The model under review builds one solid part; all positions refer to its coordinate system, in mm. Face numbers are marked on the shaded views. A direction names the side the tool comes from. Coordinates: 2 decimals unless noted, no trailing zeros. Loops run counter-clockwise (first coordinate to the right, second up) from the corner with the lowest first, then second, coordinate; pieces in that order, holes last. Notation, with made-up numbers: (13, 57.5) - (63, 57.5) arc R16 ccw to (63, 67.5) - close; hole circle Ø8 at (82, 21.5). An arc over 180 degrees is marked (long way). Answer in a Markdown table with one row per item. Add a question column.
(1) Machinability: for the marked faces 3, 4 and 5, which of the approach directions +Z, -Z, +X, -X, +Y, -Y give a long, thin tool a straight path to every point of the face, cutting with its end or side? Answer none if there is none.
(2) We need section D-D on y = -13. Write out the cut boundary in (x, z), plus the area to 3 significant figures.
(3) We need section C-C on z = 3.5. Write out the cut boundary in (x, y).
(4) We need section A-A on y = 0.75. Write out the cut boundary in (x, z), plus the area to 3 significant figures.
(5) We need section B-B on x = -0.5. Write out the cut boundary in (y, z), plus the area to 3 significant figures.
(6) For line 1 along X through (y, z) = (-14, 0); line 2 along X through (y, z) = (-1.65, 0) (3 decimals), list the stretches that pass through material, from the lowest coordinate up.
(7) For P1, Ø0.9, axis at x = -0.5, z = 2, coming from the +Y side; P2, Ø1.3, axis at x = 0.5, z = 1, coming from the +Y side; P3, Ø3, axis at y = -13, z = -3, coming from the -X side; P4, Ø0.5, axis at x = -1.5, z = 1.5, coming from the -Y side, all flat-tipped, find the tip position at first contact; note any pin that passes through.
(8) Mouldability with a two-part tool opening along Z and no side actions: class the marked faces 1 and 2 as +Z half, -Z half, draft (parallel to the pull), parting line (faces both ways), or undercut.
from build123d import *

# Parameters (mm, degrees)
SKETCH1_R           = 5
SKETCH1_R_2         = 2.6
BOSS_EXTRUDE1_DEPTH = 8
BOSS_EXTRUDE2_START = 6
SKETCH2_R           = 5
SKETCH2_R_2         = 2.175
BOSS_EXTRUDE2_DEPTH = 6
BOSS_EXTRUDE3_START = 1.5
SKETCH3_R           = 5
BOSS_EXTRUDE3_DEPTH = 1.5
BOSS_EXTRUDE4_START = 13
SKETCH4_R           = 5
BOSS_EXTRUDE4_DEPTH = 13


with BuildPart() as part:
    # Sketch1 → Boss-Extrude1 (new body)
    # profile 1 of 6: a face of its own
    with BuildSketch(Plane(origin=(0, 0, 0), x_dir=(1, 0, 0), z_dir=(0, 1, 0))):
        with Locations(Location((0, 0, 0), (0, 0, 270))):
            Circle(SKETCH1_R)
        Circle(SKETCH1_R_2, mode=Mode.SUBTRACT)
    # profile 2 of 6: a face of its own
    with BuildSketch(Plane(origin=(0, 0, 0), x_dir=(1, 0, 0), z_dir=(0, 1, 0))):
        with BuildLine():
            Line((2.111719424, 1.51678643), (2.095106807, -1.539651735))
            ThreePointArc((2.095106807, -1.539651735), (2.470554361, -0.810161188), (2.6, 0))
            ThreePointArc((2.6, 0), (2.474921262, 0.796721249), (2.111719424, 1.51678643))
        make_face()
    # profile 3 of 6: a face of its own
    with BuildSketch(Plane(origin=(0, 0, 0), x_dir=(1, 0, 0), z_dir=(0, 1, 0))):
        with BuildLine():
            ThreePointArc((-0.816872207, -2.468343533), (0.789992429, -2.477077303), (2.095106807, -1.539651735))
            Line((2.095106807, -1.539651735), (-0.816872207, -2.468343533))
        make_face()
    # profile 4 of 6: a face of its own
    with BuildSketch(Plane(origin=(0, 0, 0), x_dir=(1, 0, 0), z_dir=(0, 1, 0))):
        with BuildLine():
            ThreePointArc((-2.599961596, 0.014131536), (-2.111719424, -1.51678643), (-0.816872207, -2.468343533))
            Line((-0.816872207, -2.468343533), (-2.599961596, 0.014131536))
        make_face()
    # profile 5 of 6: a face of its own
    with BuildSketch(Plane(origin=(0, 0, 0), x_dir=(1, 0, 0), z_dir=(0, 1, 0))):
        with BuildLine():
            Line((-2.599961596, 0.014131536), (-0.789992429, 2.477077303))
            ThreePointArc((-0.789992429, 2.477077303), (-2.095106807, 1.539651735), (-2.599961596, 0.014131536))
        make_face()
    # profile 6 of 6: a face of its own
    with BuildSketch(Plane(origin=(0, 0, 0), x_dir=(1, 0, 0), z_dir=(0, 1, 0))):
        with BuildLine():
            Line((-0.789992429, 2.477077303), (2.111719424, 1.51678643))
            ThreePointArc((2.111719424, 1.51678643), (0.816872207, 2.468343533), (-0.789992429, 2.477077303))
        make_face()
    extrude(amount=BOSS_EXTRUDE1_DEPTH)

    # Sketch2 → Boss-Extrude2 (add)
    with BuildSketch(Plane.XZ.offset(BOSS_EXTRUDE2_START)):
        with Locations(Location((0, 0, 0), (0, 0, 270))):
            Circle(SKETCH2_R)
        with Locations(Location((0, 0, 0), (0, 0, 87.049070531))):
            Circle(SKETCH2_R_2, mode=Mode.SUBTRACT)
    extrude(amount=-BOSS_EXTRUDE2_DEPTH)

    # Sketch3 → Boss-Extrude3 (add)
    with BuildSketch(Plane.XZ.offset(6).offset(BOSS_EXTRUDE3_START)):
        with Locations(Location((0, 0, 0), (0, 0, 270))):
            Circle(SKETCH3_R)
    extrude(amount=-BOSS_EXTRUDE3_DEPTH)

    # Sketch4 → Boss-Extrude4 (add)
    with BuildSketch(Plane.XZ.offset(7.5).offset(BOSS_EXTRUDE4_START)):
        with Locations(Location((0, 0, 0), (0, 0, 270))):
            Circle(SKETCH4_R)
        with BuildLine():
            Line((-1.747140521, 2.5), (1.747140521, 2.5))
            ThreePointArc((1.747140521, 2.5), (0, -3.05), (-1.747140521, 2.5))
        make_face(mode=Mode.SUBTRACT)
    extrude(amount=-BOSS_EXTRUDE4_DEPTH)


solid = part.part
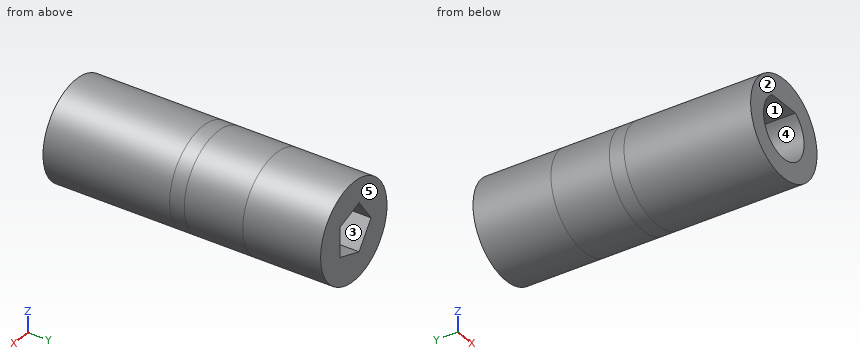
Outcome:
| question | item | result |
|---|---|---|
| 1 | face 3 | +Y |
| 1 | face 4 | -Y |
| 1 | face 5 | +Z, -Z, +X, -X, +Y |
| 2 | outline | circle Ø10 at (0, 0); hole (-1.75, 2.5) arc R3.05 ccw (long way) to (1.75, 2.5) - close |
| 2 | area | 50.6 mm² |
| 3 | outline | (-3.57, -20.5) - (3.57, -20.5) - (3.57, 8) - (-3.57, 8) - close |
| 4 | outline | circle Ø10 at (0, 0); hole (-2.6, -0.01) - (-0.79, -2.48) - (2.11, -1.52) - (2.1, 1.54) - (-0.82, 2.47) - close |
| 4 | area | 62.5 mm² |
| 5 | outline | (-20.5, -4.97) - (8, -4.97) - (8, -2.38) - (0, -2.38) - (0, -2.12) - (-6, -2.12) - (-6, 2.12) - (0, 2.12) - (0, 2.37) - (8, 2.37) - (8, 4.97) - (-20.5, 4.97) - (-20.5, 2.5) - (-7.5, 2.5) - (-7.5, -3.01) - (-20.5, -3.01) - close |
| 5 | area | 149 mm² |
| 6 | line 1 | -5 to -3.05, 3.05 to 5 |
| 6 | line 2 | -5 to -2.175, 2.175 to 5 |
| 7 | P1 | y = 8 |
| 7 | P2 | y = -6 |
| 7 | P3 | x = -4.77 |
| 7 | P4 | y = -7.5 |
| 8 | face 1 | undercut |
| 8 | face 2 | draft |
